from build123d import *

# Parameters (mm, degrees)
F0_W     = 12.7
F0_H     = 12.7
F1_DEPTH = 8.89
F2_R     = 4.1275
F3_DEPTH = 1.27
F4_R     = 3.175
F5_DEPTH = 7.62


with BuildPart() as f1:
    # F0 (on Top) → F1 (new body)
    with BuildSketch(Plane.XY):
        Rectangle(F0_W, F0_H)
    extrude(amount=F1_DEPTH)

    # F2 (on face) → F3 (join)
    with BuildSketch(Plane.XY.offset(8.89)):
        Circle(F2_R)
    extrude(amount=F3_DEPTH)

    # F4 (on face) → F5 (join)
    with BuildSketch(Plane.XY.offset(10.16)):
        Circle(F4_R)
    extrude(amount=F5_DEPTH)


solid = f1.part
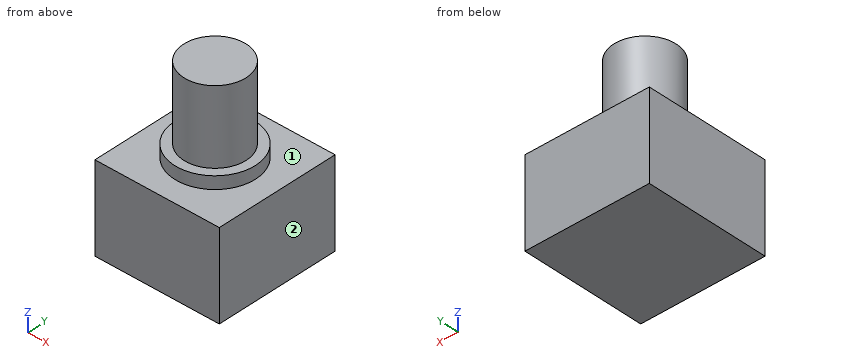
Design review of the part built by this model. Coordinates are the model's own, in mm. Face numbers are marked on the shaded views. A direction names the side the tool comes from. Give positions to 0.01 mm unless a question says otherwise; leave off trailing zeros. Order: outer loops, then holes, each group sorted by start corner. A loop starts at its lowest first (then second) coordinate and runs counter-clockwise, first axis right, second up. Notation, with made-up numbers: (31.5, 40.5) - (59.5, 40.5) arc R18 cw to (59.5, 71.5) - close; hole circle Ø4 at (63, 82). An arc over 180 degrees is marked (long way). Write item = value, one per line. Start each with the question number.
Q1. To check wall thickness, follow L1, parallel to Z at x = -2.5, y = -5.25; L2, parallel to Z at x = 0.75, y = 3.5; L3, parallel to Y at x = 1.25, z = 9.5. State the ranges of each line that lie inside material, in increasing order. Write a range as from..to.
Q2. We need section D-D on z = 9.25. State the section outline as (x, y) points (1 decimal).
Q3. We need section C-C on z = 13. State the section outline as (x, y) points (3 decimals).
Q4. Tool access review of the marked faces 1 and 2: name each direction out of +Z, -Z, +X, -X, +Y, -Y from which nothing blocks a thin tool from reaching the whole face with its end or side.
Working result:
q1.L1 = 0..8.89
q1.L2 = 0..10.16
q1.L3 = -3.93..3.93
q2.outline = circle Ø8.3 at (0, 0)
q3.outline = circle Ø6.35 at (0, 0)
q4.face_1 = +Z
q4.face_2 = +Z, -Z, +X, +Y, -Y
